from build123d import *

# Parameters (mm, degrees)
F1_DEPTH      = 5
F3_DEPTH      = 5
F3_DEPTH_BACK = 5
F4_R          = 2.5
F5_DEPTH      = 5.001
F12_W         = 57.105852
F12_H         = 43.326581
F13_DEPTH     = 5


with BuildPart() as f1:
    # F0 (on Front) → F1 (new body)
    with BuildSketch(Plane.XZ):
        with BuildLine():
            Line((0, 9.13175), (0, 7.5))
            ThreePointArc((0, 7.5), (-6.835784, -3.085784), (5.625, -4.960784))
            Line((5.625, -4.960784), (10, 0))
            Line((10, 0), (10, 10))
            Line((10, 10), (3.75, 25))
            Line((3.75, 25), (1.25, 25))
            Line((1.25, 25), (1.25, 10))
            Line((1.25, 10), (0, 9.13175))
        make_face()
    extrude(amount=F1_DEPTH)

    # F2 (on face) → F3 (join, two sides)
    with BuildSketch(Plane.XZ.offset(5)) as f3_sk:
        with BuildLine():
            Line((3.75, 25), (1.25, 25))
            Line((1.25, 25), (1.25, 23.75))
            Line((1.25, 23.75), (-1.25, 22.5))
            Line((-1.25, 22.5), (1.25, 21.25))
            Line((1.25, 21.25), (-1.25, 20))
            Line((-1.25, 20), (1.25, 18.75))
            Line((1.25, 18.75), (-1.25, 17.5))
            Line((-1.25, 17.5), (1.25, 16.25))
            Line((1.25, 16.25), (-1.25, 15))
            Line((-1.25, 15), (1.25, 13.75))
            Line((1.25, 13.75), (-1.25, 12.5))
            Line((-1.25, 12.5), (1.25, 11.25))
            Line((1.25, 11.25), (-1.25, 10))
            Line((-1.25, 10), (0, 9.375))
            Line((0, 9.375), (0, 9.13175))
            Line((0, 9.13175), (0, 8.5))
            ThreePointArc((0, 8.5), (6.667708, 5.27178), (8.270751, -1.960784))
            Line((8.270751, -1.960784), (10, 0))
            Line((10, 0), (10, 10))
            Line((10, 10), (3.75, 25))
        make_face()
        Polygon((1.25, 23.75), (1.25, 25), (-1.25, 25), align=None)
    extrude(amount=F3_DEPTH)
    extrude(f3_sk.sketch, amount=-F3_DEPTH_BACK)

    # F4 (on face) → F5 (cut, through all)
    with BuildSketch(Plane.XZ.offset(5)):
        Circle(F4_R)
    extrude(amount=-F5_DEPTH, mode=Mode.SUBTRACT)

    # F12 (on face) → F13 (cut)
    with BuildSketch(Plane.XZ):
        with Locations((-1.16475, 8.679668)):
            Rectangle(F12_W, F12_H)
    extrude(amount=F13_DEPTH, mode=Mode.SUBTRACT)


with BuildPart() as f6_1:
    # F6: copy of F1
    add(f1.part)


with BuildPart() as f8_1:
    # F8: copy of F1
    add(f1.part.moved(Location((20, 0, 0))))


with BuildPart() as f10_1:
    # F10: copy of F1
    add(f1.part)


solid = f1.part
Geometry check sheet. Reference: the model listing, model coordinates, mm. A direction names the side the tool comes from. Round coordinates to 2 decimals unless told otherwise and drop trailing zeros. Order: outer loops, then holes, each group sorted by start corner. A loop starts at its lowest first (then second) coordinate and runs counter-clockwise, first axis right, second up. Notation, with made-up numbers: (73, -38.75) - (100, -38.75) arc R16 cw to (100, -25.75) - close; hole circle Ø4 at (-16.5, -11.75). An arc over 180 degrees is marked (long way). One line per question, with ' | ' between items. Start each with the question number.
(1) Sectioned sample at D-D on x = 5. Record the cut outline in (y, z), and give its area (3 significant figures).
(2) Depth check by flat-ended pin: pin 1 Ø1 at (x, y) = (0, -7) entering from -Z. Enter the tip coordinate at first touch or a pass-through.
(3) Access from +Z, -Z, +X, -X, +Y, -Y to the whole of each face (thin tool, end or side, straight path). Record for faces 1 (the flat face through (0, -7, 9)), 2 (the flat face through (-0.017, -7.535, 21.884)), 3 (the flat face through (4, -5, 12)).
(4) Sectioned sample at C-C on z = 11.5. Record the cut outline in (x, y) (3 decimals), and give its area (3 significant figures).
(5) Thickness scan on L1, parallel to X at y = -7.2, z = 2.75; L2, parallel to X at y = -7.2, z = 4.25; L3, parallel to Z at x = 5.75, y = -7.3. Record the ranges inside material, lowest first. Write a range as [from, to].
(6) Release check for a two-part mould opening along Z. For faces 4 (the flat face through (6.919, -7.465, 17.395)), 5 (the flat face through (9.123, -7.465, -0.994)), 6 (the flat face through (0.017, -7.535, 18.134)) record: released by +Z, released by -Z, zero draft, split by the parting line, or undercut.
(7) Sectioned sample at A-A on x = -0.25. Record the cut outline in (y, z).
(8) Sectioned sample at B-B on y = -9.05. Record the cut outline in (x, z) (3 decimals), and give its area (3 significant figures).
Conclusion:
1) outline: (-10, 6.87) - (-5, 6.87) - (-5, 22) - (-10, 22) - close | area: 75.6 mm2
2) pin 1: stops at z = 8.49
3) face 1: -Z, -X, +Y, -Y | face 2: -X, +Y, -Y | face 3: +Z, -Z, +X, -X, +Y
4) outline: (0.75, -10) - (9.375, -10) - (9.375, -5) - (0.75, -5) - close | area: 43.1 mm2
5) L1: x = [8.04, 10] | L2: x = [7.36, 10] | L3: z = [6.26, 20.2]
6) face 4: released by +Z | face 5: released by -Z | face 6: undercut
7) outline: (-10, 9.5) - (-5, 9.5) - (-5, 10.5) - (-10, 10.5) - close; (-10, 12) - (-5, 12) - (-5, 13) - (-10, 13) - close; (-10, 14.5) - (-5, 14.5) - (-5, 15.5) - (-10, 15.5) - close; (-10, 17) - (-5, 17) - (-5, 18) - (-10, 18) - close; (-10, 19.5) - (-5, 19.5) - (-5, 20.5) - (-10, 20.5) - close; (-10, 22) - (-5, 22) - (-5, 23) - (-10, 23) - close; (-10, 24.5) - (-5, 24.5) - (-5, 25) - (-10, 25) - close
8) outline: (-1.25, 10) - (0, 9.375) - (0, 8.5) arc R8.5 cw to (8.271, -1.961) - (10, 0) - (10, 10) - (3.75, 25) - (-1.25, 25) - (1.25, 23.75) - (-1.25, 22.5) - (1.25, 21.25) - (-1.25, 20) - (1.25, 18.75) - (-1.25, 17.5) - (1.25, 16.25) - (-1.25, 15) - (1.25, 13.75) - (-1.25, 12.5) - (1.25, 11.25) - close | area: 148 mm2
